from build123d import *

# Parameters (mm, degrees)
CROQUIS1_R              = 5.5
SALIENTE_EXTRUIR1_DEPTH = 26.5
CROQUIS2_R              = 7.2
SALIENTE_EXTRUIR2_DEPTH = 2.3
CROQUIS3_W              = 11.5
CROQUIS3_H              = 4.45
SALIENTE_EXTRUIR3_DEPTH = 14
CORTAR_EXTRUIR1_DEPTH   = 13.37
CROQUIS6_R              = 4
CORTAR_EXTRUIR2_DEPTH   = 26.5
CROQUIS7_R              = 2.8
CORTAR_EXTRUIR3_DEPTH   = 26.37
CHAFL_N1_SIZE           = 0.9
CHAFL_N1_SIZE2          = 3.358845727
CHAFL_N2_SIZE           = 3.358845727
CHAFL_N2_SIZE_2         = 0.9
REDONDEO1_R             = 0.2
REDONDEO2_R             = 0.2
CROQUIS11_W             = 4
CROQUIS11_H             = 22.3
CORTAR_EXTRUIR4_DEPTH   = 48.550085436
CORTAR_EXTRUIR5_DEPTH   = 8.4
REDONDEO3_R             = 0.2
CHAFL_N3_SIZE           = 1
CHAFL_N3_SIZE2          = 0.577350269


with BuildPart() as part:
    # Croquis1 → Saliente-Extruir1 (new body)
    with BuildSketch(Plane(origin=(0, 0, 0), x_dir=(1, 0, 0), z_dir=(0, 1, 0))):
        with Locations(Location((0, 0, 0), (0, 0, 270))):
            Circle(CROQUIS1_R)
    extrude(amount=SALIENTE_EXTRUIR1_DEPTH)

    # Croquis2 → Saliente-Extruir2 (add)
    with BuildSketch(Plane(origin=(0, 26.5, 0), x_dir=(1, 0, 0), z_dir=(0, 1, 0))):
        with Locations(Location((0, 0, 0), (0, 0, 270))):
            Circle(CROQUIS2_R)
    extrude(amount=SALIENTE_EXTRUIR2_DEPTH)

    # Croquis3 → Saliente-Extruir3 (add)
    with BuildSketch(Plane(origin=(0, 28.8, 0), x_dir=(1, 0, 0), z_dir=(0, 1, 0))):
        Rectangle(CROQUIS3_W, CROQUIS3_H)
    extrude(amount=SALIENTE_EXTRUIR3_DEPTH)

    # Croquis4 → Cortar-Extruir1 (cut)
    with BuildSketch(Plane.XY.offset(2.225)):
        with BuildLine():
            Line((5.75, 42.8), (0, 42.8))
            ThreePointArc((0, 42.8), (4.065863992, 41.115863992), (5.75, 37.05))
            Line((5.75, 37.05), (5.75, 42.8))
        make_face()
        with BuildLine():
            Line((0, 42.8), (-5.75, 42.8))
            Line((-5.75, 42.8), (-5.75, 37.05))
            ThreePointArc((-5.75, 37.05), (-4.065863992, 41.115863992), (0, 42.8))
        make_face()
    extrude(amount=-CORTAR_EXTRUIR1_DEPTH, mode=Mode.SUBTRACT)

    # Croquis6 → Cortar-Extruir2 (cut)
    with BuildSketch(Plane.XZ):
        with Locations(Location((0, 0, 0), (0, 0, 270))):
            Circle(CROQUIS6_R)
    extrude(amount=-CORTAR_EXTRUIR2_DEPTH, mode=Mode.SUBTRACT)

    # Croquis7 → Cortar-Extruir3 (cut)
    with BuildSketch(Plane.XY.offset(2.225)):
        with Locations((0, 37.05)):
            Circle(CROQUIS7_R)
    extrude(amount=-CORTAR_EXTRUIR3_DEPTH, mode=Mode.SUBTRACT)

    # Chaflán1
    chafl_n1_edges = [part.edges().sort_by_distance(p)[0] for p in [
        (-2.8, 37.05, 2.225),
    ]]
    chafl_n1_side = [part.faces().sort_by_distance(p)[0] for p in [
        (0, 28.981176709, 2.225),
    ]]
    chamfer(chafl_n1_edges, length=CHAFL_N1_SIZE, length2=CHAFL_N1_SIZE2, reference=chafl_n1_side[0])

    # Chaflán2
    # the kernel refuses this chamfer: 3.358845727, 0.9 mm, written as the material it takes off along each edge
    with BuildSketch(Plane(origin=(0, 37.05, -2.225), x_dir=(1, 0, 0), z_dir=(0, -1, 0))) as chafl_n2_piece_1:
        Polygon((2.8, CHAFL_N2_SIZE), (2.8 + CHAFL_N2_SIZE_2, 0), (2.8, 0), align=None)
    revolve(axis=Axis((0, 37.05, -2.225), (0, 0, 1)), mode=Mode.SUBTRACT)

    # Redondeo1
    redondeo1_edges = [part.edges().sort_by_distance(p)[0] for p in [
        (-5.75, 32.925, 2.225),
        (-5.75, 32.925, -2.225),
        (0, 42.8, 2.225),
        (0, 42.8, -2.225),
        (5.75, 32.925, -2.225),
        (5.75, 32.925, 2.225),
    ]]
    fillet(redondeo1_edges, radius=REDONDEO1_R)

    # Redondeo2
    redondeo2_edges = [part.edges().sort_by_distance(p)[0] for p in [
        (-3.7, 37.05, 2.225),
        (-3.7, 37.05, -2.225),
        (-3.103813047, 37.05, 0),
    ]]
    fillet(redondeo2_edges, radius=REDONDEO2_R)

    # Croquis11 → Cortar-Extruir4 (cut, through all)
    with BuildSketch(Plane.XY.offset(12.225)):
        with Locations((0, 15.35)):
            Rectangle(CROQUIS11_W, CROQUIS11_H)
    extrude(amount=-CORTAR_EXTRUIR4_DEPTH, mode=Mode.SUBTRACT)

    # Croquis13 → Cortar-Extruir5 (cut)
    with BuildSketch(Plane.XZ):
        with BuildLine():
            Line((-2, -4.19791615), (4.520060123, 1.091584394))
            ThreePointArc((4.520060123, 1.091584394), (3.611110666, 2.929569892), (2, 4.19791615))
            Line((2, 4.19791615), (-4.520060123, -1.091584394))
            ThreePointArc((-4.520060123, -1.091584394), (-3.611110666, -2.929569892), (-2, -4.19791615))
        make_face()
    extrude(amount=-CORTAR_EXTRUIR5_DEPTH, mode=Mode.SUBTRACT)

    # Redondeo3
    redondeo3_edges = [part.edges().sort_by_distance(p)[0] for p in [
        (-2, 4.2, -4.660695766),
        (-2, 4.2, 4.293788499),
        (-2, 26.5, -4.293788499),
        (-2, 26.5, 4.293788499),
        (2, 26.5, 4.293788499),
        (2, 26.5, -4.293788499),
        (2, 4.2, -4.293788499),
        (2, 4.2, 4.660695766),
    ]]
    fillet(redondeo3_edges, radius=REDONDEO3_R)

    # Chaflán3
    chafl_n3_edges = [part.edges().sort_by_distance(p)[0] for p in [
        (0, 28.8, -7.2),
    ]]
    chafl_n3_side = [part.faces().sort_by_distance(p)[0] for p in [
        (-5.953646753, 28.8, 0),
    ]]
    chamfer(chafl_n3_edges, length=CHAFL_N3_SIZE, length2=CHAFL_N3_SIZE2, reference=chafl_n3_side[0])


solid = part.part
Source: CAD feature listing. Evaluate the final solid. Frame: model axes, mm. A direction names the side the tool comes from. Round coordinates to 2 decimals unless told otherwise and drop trailing zeros. Loops run counter-clockwise (first coordinate to the right, second up) from the corner with the lowest first, then second, coordinate; pieces in that order, holes last. Notation, with made-up numbers: M 17.25,15.25 L 22.25,15.25 A5 ccw 22.25,23.25 Z; hole C 33.5,-39 d6. An arc over 180 degrees is marked long. Answer as CSV lines item,"result".
Q1. Cut plane B-B (y = 32). Return the cut outline in (x, z) (3 decimals).
Verdict:
outline,"M -5.75,-2.025 A0.2 ccw -5.55,-2.225 L 5.55,-2.225 A0.2 ccw 5.75,-2.025 L 5.75,2.025 A0.2 ccw 5.55,2.225 L -5.55,2.225 A0.2 ccw -5.75,2.025 Z"
Q2. Reachability of faces 4 (the face through (-5.37, 13.06, -1.19)), 5 (the face through (2, 15, -4)), 6 (the face through (-5.75, 33, 0)) from +Z, -Z, +X, -X, +Y, -Y: full face, straight path, thin tool, end or side. Return the list, or none.
Verdict:
face 4,"-Y"
face 5,"+Z, -Z"
face 6,"+Z, -Z, -X, +Y"
Q3. Contact query for flat-ended pins moving along their axis: pin 1 (1.3 mm diameter, centred on x = 2.5, z = 2.5, fed in from -Y); pin 2 (1.3 mm diameter, centred on y = 18.5, z = -4, fed in from -X); pin 3 (4 mm diameter, centred on y = 4.5, z = -0.5, fed in from +X). Output: stop coordinate, or through.
Verdict:
pin 1,"stops at y = 8.4"
pin 2,"stops at x = -4.36"
pin 3,"stops at x = 5.5"
Q4. Cut plane A-A (y = 18). Return the cut outline in (x, z), plus the area to 3 significant figures.
Verdict:
outline,"M -2,-5.12 L -2,-3.46 A4 cw -2,3.46 L -2,5.12 A5.5 ccw Z; M 2,-5.12 A5.5 ccw 2,5.12 L 2,3.46 A4 cw 2,-3.46 Z"
area,"32.4 mm^2"
Q5. Cut plane C-C (x = -0.5). Count the separate pieces of the cut face and the enclosed holes in it, plus the area to 3 significant figures.
Verdict:
separate pieces,"4"
enclosed holes,"0"
area,"77.4 mm^2"
Q6. Pull-direction query (Y, two-part tool) for faces 1 (the face through (0, 33, -2.225)), 2 (the face through (0, 28.8, 3)), 3 (the face through (-2, 15, -4)); classes: +Y half, -Y half, draft (parallel to the pull), parting line (faces both ways), or undercut.
Verdict:
face 1,"draft"
face 2,"+Y half"
face 3,"undercut"
Q7. Line query: line 1 along Y through (x, z) = (-1.25, 5); line 2 along X through (y, z) = (22.5, -1.25); line 3 along Z through (x, y) = (-0.5, 33) (3 decimals). Output: solid intervals per line, ascending.
Verdict:
line 1,"y = 0 to 4.2, 26.5 to 28.8"
line 2,"x = -5.36 to -3.8, 3.8 to 5.36"
line 3,"z = -2.225 to 2.225"
